from build123d import *

# Parameters (mm, degrees)
F0_W     = 360.729664
F0_H     = 148.37706
F1_DEPTH = 25.4
F2_R     = 25.885086
F3_DEPTH = 25.4


with BuildPart() as f1:
    # F0 (on Front) → F1 (new body)
    with BuildSketch(Plane.XZ):
        Rectangle(F0_W, F0_H)
        Polygon((-148.697704, -26.601247), (-112.246476, 43.323327), (-75.345226, 47.225576), (-78.495331, 12.56507), (-49.244333, 18.759031), (-48.344307, 44.669721), (-13.243117, 51.652454), (-16.843244, 24.062283), (16.457889, 27.825298), (20.958038, 53.875219), (59.209336, 57.717167), (53.35914, 27.677407), (40.308692, -11.641144), align=None, mode=Mode.SUBTRACT)
    extrude(amount=F1_DEPTH)

    # F2 (on face) → F3 (cut)
    with BuildSketch(Plane(origin=(0, 0, 0), x_dir=(-1, 0, 0), z_dir=(0, 1, 0))):
        with Locations((-99.316008, 37.326083)):
            Circle(F2_R)
    extrude(amount=-F3_DEPTH, mode=Mode.SUBTRACT)


solid = f1.part
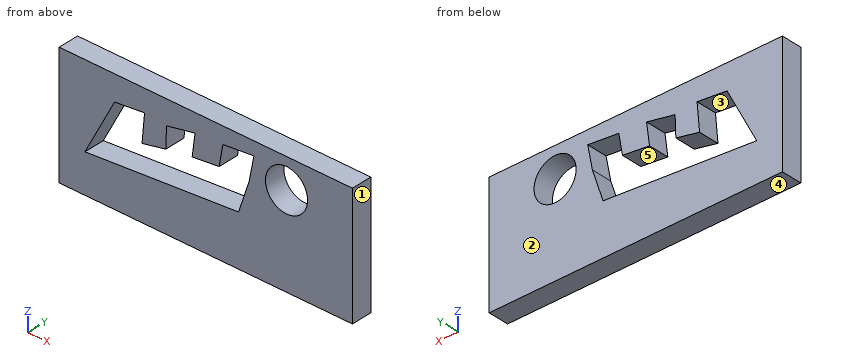
Work out the finished part from the listing and answer in its coordinate system (mm). Face numbers are marked on the shaded views. A direction names the side the tool comes from. Give positions to 0.01 mm unless a question says otherwise; leave off trailing zeros. Write each loop counter-clockwise with the first axis right and the second up, starting at its lowest first coordinate (ties: lowest second). Pieces come first, ordered by that corner, then holes. Notation, with made-up numbers: (-29.5, 75.25) - (27.5, 75.25) arc R21 cw to (27.5, 96.25) - close; hole circle Ø2 at (-11, -22). An arc over 180 degrees is marked (long way). One line per item, written item: value. Start each with the question number.
1. For a pull along X with two mould halves and no side action, classify the marked faces 1, 2 and 3 as +X half, -X half, draft (parallel to the pull), parting line (faces both ways), or undercut.
2. Find section C-C (y = -6.5). Write down the section's boundary in (x, z), then the cut area to 3 significant figures.
3. For the marked faces 4 and 5, determine the directions among +Z, -Z, +X, -X, +Y, -Y from which every point of the face is accessible in a straight line to the end or side of a thin tool.
4. Find section A-A (x = -135). Write down the section's boundary in (y, z).
5. Consider probe 1 along X at (y, z) = (-16.75, 29); probe 2 along X at (y, z) = (-18.5, 9.5); probe 3 along X at (y, z) = (-20.75, 8.5). Determine where each line is inside the solid, lowest interval first.
6. Find section B-B (z = 7). Write down the section's boundary in (x, y), then the cut area to 3 significant figures.
Geometry results:
1. face 1: +X half
1. face 2: draft
1. face 3: undercut
2. outline: (-180.36, -74.19) - (180.36, -74.19) - (180.36, 74.19) - (-180.36, 74.19) - close; hole (-148.7, -26.6) - (40.31, -11.64) - (53.36, 27.68) - (59.21, 57.72) - (20.96, 53.88) - (16.46, 27.83) - (-16.84, 24.06) - (-13.24, 51.65) - (-48.34, 44.67) - (-49.24, 18.76) - (-78.5, 12.57) - (-75.35, 47.23) - (-112.25, 43.32) - close; hole circle Ø51.77 at (99.32, 37.33)
2. area: 41,100 mm2
3. face 4: -Z, +X, -X, +Y, -Y
3. face 5: +Y, -Y
4. outline: (-25.4, -74.19) - (0, -74.19) - (0, -25.52) - (-25.4, -25.52) - close; (-25.4, -0.32) - (0, -0.32) - (0, 74.19) - (-25.4, 74.19) - close
5. probe 1: -180.36 to -119.71, -77 to -48.89, -16.2 to 16.66, 53.62 to 74.81, 123.83 to 180.36
5. probe 2: -180.36 to -129.88, 47.33 to 180.36
5. probe 3: -180.36 to -130.4, 46.99 to 180.36
6. outline: (-180.36, -25.4) - (-131.18, -25.4) - (-131.18, 0) - (-180.36, 0) - close; (46.5, -25.4) - (180.36, -25.4) - (180.36, 0) - (46.5, 0) - close
6. area: 4,650 mm2
